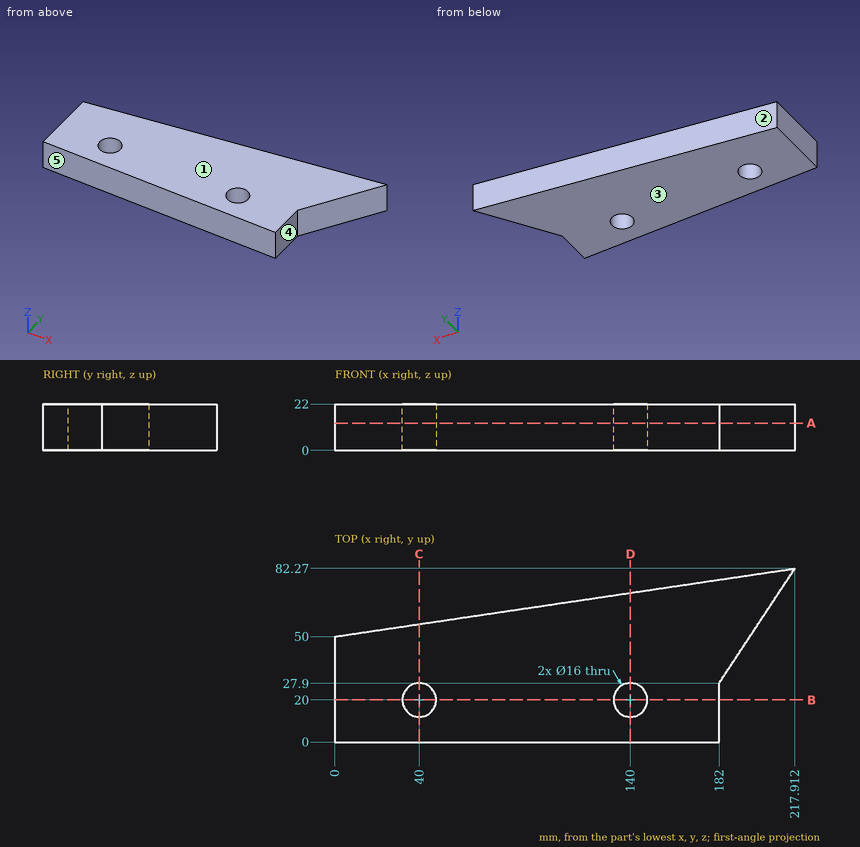
Check sheet for the drawn part. Datum: minimum x, y, z corner. Units: mm. A direction names the side the tool comes from. Round coordinates to 2 decimals unless told otherwise and drop trailing zeros. Loops run counter-clockwise (first coordinate to the right, second up) from the corner with the lowest first, then second, coordinate; pieces in that order, holes last. Notation, with made-up numbers: (73, 45) -> (115, 45) arc R8 cw to (115, 56) -> close; hole circle Ø7 at (-1.75, 12). An arc over 180 degrees is marked (long way). Put each result on its own line as item: value. Start each with the question number.
1. Section check B-B (y = 20). Enter the section's corners in (x, z).
2. Access from +Z, -Z, +X, -X, +Y, -Y to the whole of each face (thin tool, end or side, straight path). Record for the marked faces 4 and 5.
3. Section check C-C (x = 40). Enter the section's corners in (y, z).
4. Gauge pin test, flat ends, axial feed: pin 1 (2 mm diameter, centred on y = 20.5, z = 5, fed in from +X); pin 2 (6 mm diameter, centred on y = 28, z = 11.5, fed in from +X). Record the tip position at first contact, or that the pin passes through.
5. Section check D-D (x = 140). Enter the section's corners in (y, z), plus the area to 3 significant figures.
6. Draft check along Z on the marked faces 1, 2 and 3. Enter one of: +Z half, -Z half, draft (parallel to the pull), parting line (faces both ways), or undercut.
7. Scan lines: probe 1 along Y at (x, z) = (40, 11.25); probe 2 along X at (y, z) = (5.5, 6); probe 3 along Y at (x, z) = (140, 13.5). Record each from-to range of solid material in increasing order.
8. Section check A-A (z = 13). Enter the section's corners in (x, y).
Findings:
1. outline: (0, 0) -> (32, 0) -> (32, 22) -> (0, 22) -> close; (48, 0) -> (132, 0) -> (132, 22) -> (48, 22) -> close; (148, 0) -> (182, 0) -> (182, 22) -> (148, 22) -> close
2. face 4: +Z, -Z, +X, -Y
2. face 5: +Z, -Z, +X, -X, -Y
3. outline: (0, 0) -> (12, 0) -> (12, 22) -> (0, 22) -> close; (28, 0) -> (55.92, 0) -> (55.92, 22) -> (28, 22) -> close
4. pin 1: stops at x = 182
4. pin 2: stops at x = 184.05
5. outline: (0, 0) -> (12, 0) -> (12, 22) -> (0, 22) -> close; (28, 0) -> (70.73, 0) -> (70.73, 22) -> (28, 22) -> close
5. area: 1,200 mm^2
6. face 1: +Z half
6. face 2: draft
6. face 3: -Z half
7. probe 1: y = 0 to 12, 28 to 55.92
7. probe 2: x = 0 to 182
7. probe 3: y = 0 to 12, 28 to 70.73
8. outline: (0, 0) -> (182, 0) -> (182, 27.9) -> (217.91, 82.27) -> (0, 50) -> close; hole circle Ø16 at (40, 20); hole circle Ø16 at (140, 20)
